```python
from build123d import *

# Parameters (mm, degrees)
BOSS_EXTRUDE1_DEPTH            = 30
CUT_EXTRUDE1_DEPTH             = 50
FILLET1_R                      = 1
CBORE_FOR_M3_SHCS1_D           = 3.4
CBORE_FOR_M3_SHCS1_DEPTH       = 5
CBORE_FOR_M3_SHCS1_CBORE_D     = 6.5
CBORE_FOR_M3_SHCS1_CBORE_DEPTH = 3
CBORE_FOR_M3_SHCS1_TIP         = 1.021463052


with BuildPart() as part:
    # Sketch1 → Boss-Extrude1 (new body, symmetric)
    with BuildSketch(Plane(origin=(0, 0, 0), x_dir=(1, 0, 0), z_dir=(0, 1, 0))):
        with BuildLine():
            Line((-15, -28.348661632), (15, -28.348661632))
            ThreePointArc((15, -28.348661632), (34.752533521, 3), (15, 34.348661632))
            Line((15, 34.348661632), (-15, 34.348661632))
            ThreePointArc((-15, 34.348661632), (-34.752533521, 3), (-15, -28.348661632))
        make_face()
        with BuildLine():
            Line((-10, -23.348661632), (10, -23.348661632))
            ThreePointArc((10, -23.348661632), (0, 25.4), (-10, -23.348661632))
        make_face(mode=Mode.SUBTRACT)
    extrude(amount=BOSS_EXTRUDE1_DEPTH, both=True)

    # Sketch4 → Cut-Extrude1 (cut)
    with BuildSketch(Plane(origin=(0, 30, 0), x_dir=(1, 0, 0), z_dir=(0, 1, 0))):
        Polygon((-10, 34.348661632), (-10, 31.348661632), (-13.5, 31.348661632), (-13.5, 27.848661632), (13.5, 27.848661632), (13.5, 31.348661632), (10, 31.348661632), (10, 34.348661632), align=None)
    extrude(amount=-CUT_EXTRUDE1_DEPTH, mode=Mode.SUBTRACT)

    # Fillet1
    fillet1_edges = [part.edges().sort_by_distance(p)[0] for p in [
        (10, 5, -31.348661632),
        (13.5, 5, -31.348661632),
        (13.5, 5, -27.848661632),
        (-13.5, 5, -27.848661632),
        (-13.5, 5, -31.348661632),
        (-10, 5, -31.348661632),
    ]]
    fillet(fillet1_edges, radius=FILLET1_R)

    # CBORE for M3 SHCS1
    with Locations(Plane.XY.offset(28.348661632)):
        with Locations((0, 0), (0, 15), (0, -15)):
            CounterBoreHole(CBORE_FOR_M3_SHCS1_D / 2, CBORE_FOR_M3_SHCS1_CBORE_D / 2, CBORE_FOR_M3_SHCS1_CBORE_DEPTH, depth=CBORE_FOR_M3_SHCS1_DEPTH)
            with Locations((0, 0, -(CBORE_FOR_M3_SHCS1_DEPTH + CBORE_FOR_M3_SHCS1_TIP / 2))):  # 118° drill point
                Cone(0, CBORE_FOR_M3_SHCS1_D / 2, CBORE_FOR_M3_SHCS1_TIP, mode=Mode.SUBTRACT)


solid = part.part
```
Part model, mm, in its own coordinate system. A direction names the side the tool comes from. Give positions to 0.01 mm unless a question says otherwise; leave off trailing zeros. Loops run counter-clockwise (first coordinate to the right, second up) from the corner with the lowest first, then second, coordinate; pieces in that order, holes last. Notation, with made-up numbers: M 30.5,73.5 L 70.5,73.5 A16 cw 70.5,78.5 Z; hole C 48.25,-35 d8. An arc over 180 degrees is marked long. Return JSON: item names as keys, results as strings.
1) Pull direction X, two halves, no side cores. Call faces 6 (the face through (-34.75, 0.42, -3.55)), 7 (the face through (-4, 0, 28.349)), 8 (the face through (-0.423, -11.778, 26.87)): released by +X, released by -X, zero draft, split by the parting line, or undercut.
Calculated:
{"face 6": "released by -X", "face 7": "zero draft", "face 8": "undercut"}
2) Saw through at B-B, the plane x = 0. Count the separate pieces of the cut face and the enclosed holes in it, then the cut area to 3 significant figures.
Calculated:
{"separate pieces": "5", "enclosed holes": "0", "area": "433 mm2"}
3) Drill centre lines: line 1 (Y direction, x = 0, z = 27); line 2 (Y direction, x = 0, z = 24); line 3 (Z direction, x = 1, y = 13). Where is each one in solid material? Low to high.
Calculated:
{"line 1": "y = -30 to -18.25, -11.75 to -3.25, 3.25 to 11.75, 18.25 to 30", "line 2": "y = -30 to -16.7, -13.3 to -1.7, 1.7 to 13.3, 16.7 to 30", "line 3": "z = -27.85 to -25.38, 23.35 to 25.35"}
4) Flat gauge pins, fed straight in: pin 1 Ø6 at (x, y) = (2.5, 3) entering from -Z; pin 2 Ø8 at (y, z) = (-0.5, 15) entering from +X; pin 3 Ø1.2 at (y, z) = (16.5, -29.5) entering from -X. Where does each tip first touch, or does it go through?
Calculated:
{"pin 1": "stops at z = -27.85", "pin 2": "stops at x = 31.81", "pin 3": "stops at x = -23.17"}
5) 3-axis set-ups, long thin cutter, end or side, ignore diameter. For faces 1 (the face through (0, -20, -31)), 2 (the face through (1.4, -16.4, 25.349)), 3 (the face through (2, 0, 23.349)), 4 (the face through (10, 5, -33)), 5 (the face through (-8.2, -30, -24.3)): which of +Z, -Z, +X, -X, +Y, -Y reach the whole face in a straight line?
Calculated:
{"face 1": "+Y", "face 2": "+Z", "face 3": "+Y, -Y", "face 4": "-Z, +Y", "face 5": "+Z, -Z, +X, -X, -Y"}
6) Saw through at D-D, the plane x = -22.5. List the corners of the cut face in (y, z), then the cut area to 3 significant figures.
Calculated:
{"outline": "M -30,-29.49 L 30,-29.49 L 30,-11.79 L -30,-11.79 Z; M -30,11.79 L 30,11.79 L 30,23.49 L -30,23.49 Z", "area": "1,760 mm2"}
7) Saw through at C-C, the plane z = -18. List the corners of the cut face in (x, y).
Calculated:
{"outline": "M -31.35,-30 L -17.92,-30 L -17.92,30 L -31.35,30 Z; M 17.92,-30 L 31.35,-30 L 31.35,30 L 17.92,30 Z"}
8) Saw through at A-A, the plane y = -5. List the corners of the cut face in (x, z).
Calculated:
{"outline": "M -15,-34.35 L -10,-34.35 L -10,-32.35 A1 ccw -11,-31.35 L -12.5,-31.35 A1 cw -13.5,-30.35 L -13.5,-28.85 A1 cw -12.5,-27.85 L 12.5,-27.85 A1 cw 13.5,-28.85 L 13.5,-30.35 A1 cw 12.5,-31.35 L 11,-31.35 A1 ccw 10,-32.35 L 10,-34.35 L 15,-34.35 A34.75 ccw 15,28.35 L -15,28.35 A34.75 ccw Z; hole M -10,23.35 A25.4 ccw long 10,23.35 Z"}
